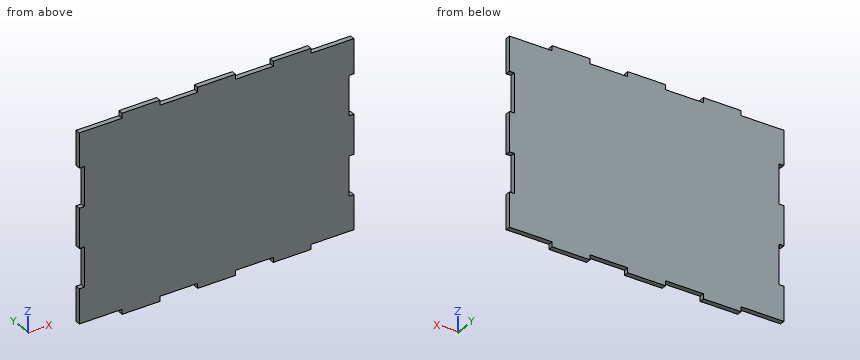
Autodesk Inventor part; units mm, degrees
ref_plane "YZ Plane" through (0, 0, 0) normal (1, 0, 0) x (0, 1, 0)
ref_plane "XZ Plane" through (0, 0, 0) normal (0, 1, 0) x (-1, 0, 0)
ref_plane "XY Plane" through (0, 0, 0) normal (0, 0, 1) x (1, 0, 0)
sketch "Sketch1" plane through (0, 0, 0) normal (0, 1, 0) x (-1, 0, 0)
  line L0 (-11.4286, -54) -> (-11.4286, -57)
  line L1 (-11.4286, -57) -> (11.4286, -57)
  line L2 (11.4286, -57) -> (11.4286, -54)
  line L3 (-57.1429, -54) -> (-57.1429, -57)
  line L4 (-57.1429, -57) -> (-34.2857, -57)
  line L5 (-34.2857, -57) -> (-34.2857, -54)
  line L6 (57.1429, -54) -> (57.1429, -57)
  line L7 (57.1429, -57) -> (34.2857, -57)
  line L8 (34.2857, -57) -> (34.2857, -54)
  line L9 (34.2857, 60) -> (34.2857, 63)
  line L10 (34.2857, 63) -> (57.1429, 63)
  line L11 (57.1429, 63) -> (57.1429, 60)
  line L12 (-11.4286, 60) -> (-11.4286, 63)
  line L13 (-11.4286, 63) -> (11.4286, 63)
  line L14 (11.4286, 63) -> (11.4286, 60)
  line L15 (-57.1429, 60) -> (-57.1429, 63)
  line L16 (-57.1429, 63) -> (-34.2857, 63)
  line L17 (-34.2857, 63) -> (-34.2857, 60)
  line L18 (80, 60) -> (83, 60)
  line L19 (83, -54) -> (80, -54)
  line L20 (-80, 60) -> (-83, 60)
  line L21 (-83, -54) -> (-80, -54)
  line L22 (80, -54) -> (80, -54)
  line L23 (80, 60) -> (80, 60)
  line L24 (57.1429, -54) -> (80, -54)
  line L25 (11.4286, -54) -> (34.2857, -54)
  line L26 (-80, -54) -> (-57.1429, -54)
  line L27 (-34.2857, -54) -> (-11.4286, -54)
  line L28 (-80, 60) -> (-80, 60)
  line L29 (-80, -54) -> (-80, -54)
  line L30 (-57.1429, 60) -> (-80, 60)
  line L31 (-11.4286, 60) -> (-34.2857, 60)
  line L32 (80, 60) -> (57.1429, 60)
  line L33 (34.2857, 60) -> (11.4286, 60)
  line L34 (83, -33) -> (80, -33)
  line L35 (80, -33) -> (80, -9)
  line L36 (80, -9) -> (83, -9)
  line L37 (83, 39) -> (80, 39)
  line L38 (80, 39) -> (80, 15)
  line L39 (80, 15) -> (83, 15)
  line L40 (-83, 39) -> (-80, 39)
  line L41 (-80, 39) -> (-80, 15)
  line L42 (-80, 15) -> (-83, 15)
  line L43 (-83, -9) -> (-80, -9)
  line L44 (-80, -9) -> (-80, -33)
  line L45 (-80, -33) -> (-83, -33)
  line L46 (83, -33) -> (83, -54)
  line L47 (83, 60) -> (83, 39)
  line L48 (83, 15) -> (83, -9)
  line L49 (-83, 60) -> (-83, 39)
  line L50 (-83, 15) -> (-83, -9)
  line L51 (-83, -33) -> (-83, -54)
  point P0 (0, 0)
  dimension "d40" = 160
  dimension "d47" = 22.8571
  dimension "d48" = 22.8571
  dimension "d49" = 3
  dimension "d50" = 3
  dimension "d51" = 3
  dimension "d52" = 3
  dimension "d53" = 3
  dimension "d54" = 3
  dimension "d55" = 80
  dimension "d56" = 60
  dimension "d57" = 114
  dimension "d58" = 0
  dimension "d59" = 0
  dimension "d61" = 24
  dimension "d62" = 24
  dimension "d63" = 24
  dimension "d64" = 3
extrude "Extrusion1" add sketch "Sketch1" along normal blind 3
equation "\"d40\" = shelfW"
equation "\"d47\" = 0.142857 * shelfW + 2 * tol"
equation "\"d48\" = 0.142857 * shelfW - 2 * tol"
equation "\"d49\" = tt"
equation "\"d50\" = tt"
equation "\"d51\" = tt"
equation "\"d52\" = tt"
equation "\"d53\" = tt"
equation "\"d54\" = tt"
equation "\"d57\" = -2 * tt + ht"
equation "\"d61\" = 0.2 * ht - tol"
equation "\"d62\" = 0.2 * ht + 2 * tol"
equation "\"d63\" = 0.2 * ht - 2 * tol"
equation "\"d64\" = tt"
equation "\"d31\" = tt"
equation "\"d4\" = tt"
equation "\"tt\" = 3"
equation "\"tol\" = 0"
equation "\"tiroir\" = 1"
equation "\"nHoles\" = 4"
equation "\"shelfW\" = 160"
equation "\"shelfH\" = 35"
equation "\"d43\" = 0.5 * shelfH"
properties part number "base"
Source: CAD feature listing. Evaluate the final solid. Frame: model axes, mm. Give positions to 0.01 mm unless a question says otherwise; leave off trailing zeros. Write each loop counter-clockwise with the first axis right and the second up, starting at its lowest first coordinate (ties: lowest second). Pieces come first, ordered by that corner, then holes. Notation, with made-up numbers: M -15,-35 L -1,-35 A19 ccw -1,-11 Z; hole C 4.25,14.5 d5. An arc over 180 degrees is marked long. Return JSON: item names as keys, results as strings. Group by question number.
1) Cut plane A-A, the plane x = -70. Output: boundary loops of the cut face in (y, z), plus the area to 3 significant figures.
2) Material intervals for line 1 along X through (y, z) = (1.65, -29); line 2 along Z through (x, y) = (25, 2.75), sorted ascending. Write a range as [from, to].
3) Pin query (flat end, axial travel): P1, Ø1.5, axis at y = 2, z = 23, coming from the -X side; P2, Ø1.5, axis at x = -82, y = 2, coming from the -Z side; P3, Ø1.5, axis at x = -65.5, z = -42, coming from the -Y side; P4, Ø0.9, axis at x = 67.5, y = 1, coming from the +Z side. Return the tip coordinate at first contact, or that it passes through.
4) Cut plane B-B, the plane z = 27.5. Output: boundary loops of the cut face in (x, y).
Recorded:
{
 "1": {"outline": "M 0,-54 L 3,-54 L 3,60 L 0,60 Z", "area": "342 mm²"},
 "2": {"line 1": "x = [-80, 80]", "line 2": "z = [-54, 60]"},
 "3": {"P1": "stops at x = -80", "P2": "stops at z = -54", "P3": "stops at y = 0", "P4": "stops at z = 60"},
 "4": {"outline": "M -80,0 L 80,0 L 80,3 L -80,3 Z"}
}
